The listing builds one solid part. Answer for the finished solid, in the listing's coordinates (mm). Face numbers are marked on the shaded views. A direction names the side the tool comes from. Round coordinates to 2 decimals unless told otherwise and drop trailing zeros. Loops run counter-clockwise (first coordinate to the right, second up) from the corner with the lowest first, then second, coordinate; pieces in that order, holes last. Notation, with made-up numbers: M 11.25,24.25 L 37.25,24.25 A20 ccw 37.25,32.25 Z; hole C 44.25,-18 d5. An arc over 180 degrees is marked long. Put each result on its own line as item: value. Start each with the question number.
(1) Section D-D, the plane y = -17.5 is taken. Determine the outline of the cut face in (x, z).
(2) Section C-C, the plane x = -3 is taken. Determine the outline of the cut face in (y, z), then the cut area to 3 significant figures.
(3) Which of the six approach directions +Z, -Z, +X, -X, +Y, -Y give full straight-line access (tool end or side, diameter ignored) to the marked faces 4, 5 and 6?
(4) Section A-A, the plane z = 10 is taken. Determine the outline of the cut face in (x, y).
(5) Determine the mould class of the marked faces 1, 2 and 3 for opening direction Y: released by +Y, released by -Y, zero draft, split by the parting line, or undercut.
(6) Flat-ended cylindrical pins translate along their axes: P1, Ø7.5, axis at x = 44.5, y = -125.5, coming from the +Z side; P2, Ø7.5, axis at y = -108.5, z = 39, coming from the +X side; P3, Ø10, axis at y = -72.5, z = 62, coming from the -X side; P4, Ø8, axis at x = 35.5, y = -46, coming from the -Z side. Find the tip coordinate at first contact, or state that the pin passes through.
(7) Section B-B, the plane y = -38.1 is taken. Determine the outline of the cut face in (x, z).
(8) Straight lines are drawn through the part: line 1 (Y direction, x = 38.1, z = 26.5); line 2 (Y direction, x = 38, z = 51); line 3 (X direction, y = -38, z = 28). For each, find the intervals that lie inside material, in ascending order.
```python
from build123d import *

# Parameters (mm, degrees)
F0_W      = 76.2
F0_H      = 76.2
F1_DEPTH  = 76.2
F3_D      = 25.4
F4_W      = 25.4
F4_H      = 25.4
F5_DEPTH  = 76.2
F10_DEPTH = 12.7
F12_DEPTH = 12.7


# Not quite as in the source:
# - the program builds the solid bodies; features that only make, move or delete a surface that nothing else refers to are left out


with BuildPart() as f1:
    # F0 (on Front) → F1 (new body)
    with BuildSketch(Plane.XZ):
        with Locations((38.1, 38.1)):
            Rectangle(F0_W, F0_H)
    extrude(amount=F1_DEPTH)

    # F3 (through all)
    with Locations(Plane.XY.offset(76.2)):
        with Locations((38.1, -38.1)):
            Hole(F3_D / 2)

    # F4 (on face) → F5 (join)
    with BuildSketch(Plane.XZ.offset(76.2)):
        with Locations((44.375465405, 43.5601483703)):
            Rectangle(F4_W, F4_H)
    extrude(amount=F5_DEPTH)

    # F9 (on face) → F10 (join)
    with BuildSketch(Plane(origin=(0, 0, 0), x_dir=(0, -1, 0), z_dir=(-1, 0, 0))):
        Polygon((52.085519187, 37.4724815469), (45.6362065152, 49.8980556745), (31.6506873282, 50.5255741276), (24.114480813, 38.7275184531), (30.5637934848, 26.3019443255), (44.5493126718, 25.6744258724), align=None)
    extrude(amount=F10_DEPTH)

    # F11 (on face) → F12 (join)
    with BuildSketch(Plane(origin=(0, 0, 0), x_dir=(-1, 0, 0), z_dir=(0, 1, 0))):
        with BuildLine():
            add(Edge.make_bspline(
                [(-48.0585680543, 49.9470105327), (-70.7842466593, 26.0252415357), (-45.6101675869, 24.8654493741), (-20.4360885145, 23.7056572126), (-22.884488982, 48.7872183711), (-25.3328894494, 73.8687795297), (-48.0585680543, 49.9470105327)],
                knots=[4.7123889804, 4.7123889804, 4.7123889804, 6.8067840828, 6.8067840828, 8.9011791852, 8.9011791852, 10.9955742876, 10.9955742876, 10.9955742876], degree=2, weights=[1, 0.5, 1, 0.5, 1, 0.5, 1]))
        make_face()
    extrude(amount=F12_DEPTH)


solid = f1.part
```
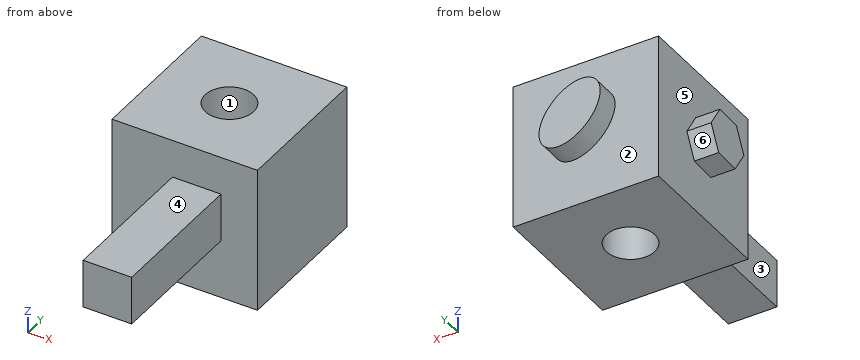
Recorded:
1. outline: M 0,0 L 76.2,0 L 76.2,76.2 L 0,76.2 Z
2. outline: M -52.09,37.47 L -44.55,25.67 L -30.56,26.3 L -24.11,38.73 L -31.65,50.53 L -45.64,49.9 Z
2. area: 509 mm²
3. face 4: +Z, +X, -X, -Y
3. face 5: -X
3. face 6: -Z, -X, +Y
4. outline: M 0,-76.2 L 76.2,-76.2 L 76.2,0 L 0,0 Z; hole C 38.1,-38.1 d25.4
5. face 1: undercut
5. face 2: released by +Y
5. face 3: zero draft
6. P1: stops at z = 56.26
6. P2: stops at x = 57.08
6. P3: stops at x = 0
6. P4: passes through
7. outline: M -12.7,25.96 L 0,25.96 L 0,0 L 25.4,0 L 25.4,76.2 L 0,76.2 L 0,50.24 L -12.7,50.24 Z; M 50.8,0 L 76.2,0 L 76.2,76.2 L 50.8,76.2 Z
8. line 1: y = -76.2 to -50.8, -25.4 to 12.7
8. line 2: y = -152.4 to -50.8, -25.4 to 12.7
8. line 3: x = -12.7 to 25.4, 50.8 to 76.2
